Model file for the job. Use its own axes, mm. A direction names the side the tool comes from. Give positions to 0.01 mm unless a question says otherwise; leave off trailing zeros. Loops run counter-clockwise (first coordinate to the right, second up) from the corner with the lowest first, then second, coordinate; pieces in that order, holes last. Notation, with made-up numbers: (-16.75, 4) - (-7.75, 4) arc R34 ccw to (-7.75, 38) - close; hole circle Ø9 at (-16.75, 7). An arc over 180 degrees is marked (long way). Use a Markdown table: item, result.
from build123d import *

# Parameters (mm, degrees)
F1_W      = 70
F1_H      = 80
F4_DEPTH  = 5
F5_W      = 55
F5_H      = 77
F7_DEPTH  = 22
F6_W      = 3.6
F6_H      = 3.6
F8_DEPTH  = 22
F3_R      = 0.889
F3_R_2    = 1.143
F3_R_3    = 2.9
F9_DEPTH  = 22.001
F10_W     = 4
F10_H     = 10
F11_DEPTH = 3
F12_W     = 10
F12_H     = 4
F12_W_2   = 4
F12_H_2   = 8
F13_DEPTH = 5
F14_W     = 8
F14_H     = 20
F15_DEPTH = 4


with BuildPart() as f4:
    # F1 (on Front) → F4 (new body)
    with BuildSketch(Plane.XZ):
        with Locations((6.625, 7.5)):
            Rectangle(F1_W, F1_H)
    extrude(amount=F4_DEPTH)

    # F5 (on Front) → F7 (join)
    with BuildSketch(Plane.XZ):
        Polygon((35.625, 47.5), (-22.375, 47.5), (-22.375, -32.5), (35.625, -32.5), (35.625, -29.5), align=None)
        with Locations((6.625, 7.5)):
            Rectangle(F5_W, F5_H, mode=Mode.SUBTRACT)
    extrude(amount=F7_DEPTH)

    # F6 (on Front) → F8 (join)
    with BuildSketch(Plane.XZ):
        with Locations((-20.575, 45.7)):
            Rectangle(F6_W, F6_H)
        with Locations((33.825, 45.7)):
            Rectangle(F6_W, F6_H)
        Polygon((8.425, -32.5), (8.425, -28.9), (4.825, -28.9), (4.825, -30.7), (4.825, -32.5), align=None)
    extrude(amount=F8_DEPTH)

    # F3 (on Front) → F9 (cut, through all)
    with BuildSketch(Plane.XZ):
        with Locations((-25.875, 23.5)):
            Circle(F3_R)
        with Locations((-25.875, 11.5)):
            Circle(F3_R)
        with Locations((-8.875, 23.5)):
            Circle(F3_R)
        with Locations((-8.875, 11.5)):
            Circle(F3_R)
        with Locations((-8.875, -13.5)):
            Circle(F3_R)
        with Locations((-25.875, -13.5)):
            Circle(F3_R)
        with Locations((-25.875, -25.5)):
            Circle(F3_R)
        with Locations((-8.875, -25.5)):
            Circle(F3_R)
        with Locations((6.625, -30.7)):
            Circle(F3_R)
        with Locations((-25.375, -29.5)):
            Circle(F3_R_2)
        with Locations((6.625, 2.5)):
            Circle(F3_R_3)
        with Locations((-25.375, 44.5)):
            Circle(F3_R_2)
        with Locations((22.125, 23.5)):
            Circle(F3_R)
        with Locations((22.125, 11.5)):
            Circle(F3_R)
        with Locations((39.125, 23.5)):
            Circle(F3_R)
        with Locations((38.625, 44.5)):
            Circle(F3_R_2)
        with Locations((22.125, -13.5)):
            Circle(F3_R)
        with Locations((22.125, -25.5)):
            Circle(F3_R)
        with Locations((39.125, -13.5)):
            Circle(F3_R)
        with Locations((39.125, -25.5)):
            Circle(F3_R)
        with Locations((38.625, -29.5)):
            Circle(F3_R_2)
        with Locations((39.125, 11.5)):
            Circle(F3_R)
        with Locations((-20.575, 45.7)):
            Circle(F3_R)
        with Locations((33.825, 45.7)):
            Circle(F3_R)
    extrude(amount=F9_DEPTH, mode=Mode.SUBTRACT)

    # F10 (on face) → F11 (cut)
    with BuildSketch(Plane.XZ.offset(5)):
        with Locations((-21.875, 17.5)):
            Rectangle(F10_W, F10_H)
        with Locations((-21.875, -19.5)):
            Rectangle(F10_W, F10_H)
        with Locations((35.125, -19.5)):
            Rectangle(F10_W, F10_H)
        with Locations((35.125, 17.5)):
            Rectangle(F10_W, F10_H)
    extrude(amount=F11_DEPTH, mode=Mode.SUBTRACT)

    # F12 (on face) → F13 (cut)
    with BuildSketch(Plane.XZ.offset(22)):
        with Locations((6.625, 45.5)):
            Rectangle(F12_W, F12_H)
        with Locations((33.625, 2.5)):
            Rectangle(F12_W_2, F12_H_2)
        with Locations((-20.375, 2.5)):
            Rectangle(F12_W_2, F12_H_2)
    extrude(amount=-F13_DEPTH, mode=Mode.SUBTRACT)

    # F14 (on face) → F15 (cut)
    with BuildSketch(Plane.XZ.offset(5)):
        Polygon((-20.875, 17.5), (-20.875, 7.5), (-12.875, 7.5), (-12.875, 27.5), (-20.875, 27.5), align=None)
        with Locations((-16.875, -19.5)):
            Rectangle(F14_W, F14_H)
        Polygon((34.125, 17.5), (34.125, 27.5), (26.125, 27.5), (26.125, 7.5), (34.125, 7.5), align=None)
        with Locations((30.125, -19.5)):
            Rectangle(F14_W, F14_H)
    extrude(amount=-F15_DEPTH, mode=Mode.SUBTRACT)


solid = f4.part
(1) Slice it at D-D, the plane z = 2.5. Write the cut outline in (x, y) (3 decimals).
Computed:
| item | result |
|---|---|
| outline | (-28.375, -5) - (-22.375, -5) - (-22.375, -17) - (-20.875, -17) - (-20.875, -5) - (3.725, -5) - (3.725, 0) - (-28.375, 0) - close; (9.525, -5) - (34.125, -5) - (34.125, -17) - (35.625, -17) - (35.625, -5) - (41.625, -5) - (41.625, 0) - (9.525, 0) - close |
(2) Pin check, flat tips, straight feed: P1, Ø2, axis at y = -12.5, z = 34, coming from the -X side (3 decimals); P2, Ø3, axis at x = -25.875, z = -25.5, coming from the -Y side; P3, Ø3, axis at y = -17, z = 21, coming from the +X side (3 decimals). Stop position of each tip, or through.
Computed:
| item | result |
|---|---|
| P1 | x = -22.375 |
| P2 | y = -5 |
| P3 | x = 35.625 |
(3) Drill centre lines: probe 1 along X at (y, z) = (-12, 27.5) (3 decimals); probe 2 along Z at (x, y) = (5, -13.75); probe 3 along Z at (x, y) = (14.5, -16.25). Where is each one in solid material? Low to high. Write a range as [from, to].
Computed:
| item | result |
|---|---|
| probe 1 | [-22.375, -20.875], [34.125, 35.625] |
| probe 2 | [-32.5, -28.9], [46, 47.5] |
| probe 3 | [-32.5, -31], [46, 47.5] |
(4) Slice it at A-A, the plane z = 11.5. Count the separate pieces of the cut face and the enclosed holes in it, plus the area to 3 significant figures.
Computed:
| item | result |
|---|---|
| separate pieces | 5 |
| enclosed holes | 0 |
| area | 301 mm² |
(5) Slice it at C-C, the plane x = -1. Write the cut outline in (y, z), plus the area to 3 significant figures.
Computed:
| item | result |
|---|---|
| outline | (-22, -32.5) - (0, -32.5) - (0, 47.5) - (-22, 47.5) - (-22, 46) - (-5, 46) - (-5, -31) - (-22, -31) - close |
| area | 451 mm² |
(6) Mould opens along Z. For faces 4 (the flat face through (-17, -3, -9.5)), 5 (the flat face through (-21.1, -22, 33.2)) say: pulls with the +Z half, pulls with the -Z half, needs draft (parallel to the pull), parting line crosses it, or undercut.
Computed:
| item | result |
|---|---|
| face 4 | undercut |
| face 5 | needs draft |
(7) 3-axis set-ups, long thin cutter, end or side, ignore diameter. For faces 1 (the flat face through (-22.375, -13, 8)), 2 (the flat face through (26.125, -3, -20)), 3 (the cylindrical face through (22.6, -2.46, 24.25)): which of +Z, -Z, +X, -X, +Y, -Y reach the whole face in a straight line?
Computed:
| item | result |
|---|---|
| face 1 | +Z, -Z, -X, -Y |
| face 2 | -Y |
| face 3 | +Y, -Y |
(8) Slice it at B-B, the plane y = -13.25. Write the cut outline in (x, z) (3 decimals).
Computed:
| item | result |
|---|---|
| outline | (-22.375, -32.5) - (35.625, -32.5) - (35.625, 47.5) - (-22.375, 47.5) - close; hole circle Ø1.778 at (-20.575, 45.7); hole (-20.875, -31) - (4.825, -31) - (4.825, -28.9) - (8.425, -28.9) - (8.425, -31) - (34.125, -31) - (34.125, 43.9) - (32.025, 43.9) - (32.025, 46) - (-18.775, 46) - (-18.775, 43.9) - (-20.875, 43.9) - close; hole circle Ø1.778 at (6.625, -30.7); hole circle Ø1.778 at (33.825, 45.7) |
